Read the model definition and answer for the solid it produces. Units are mm, in the model's axes. Give positions to 0.01 mm unless a question says otherwise; leave off trailing zeros. Write each loop counter-clockwise with the first axis right and the second up, starting at its lowest first coordinate (ties: lowest second). Pieces come first, ordered by that corner, then holes. Notation, with made-up numbers: M 58,-17 L 74,-17 A22 ccw 74,22 Z; hole C 25,33.5 d4. An arc over 180 degrees is marked long. Use a Markdown table: item, result. Add a question column.
Item 1: The mould has two halves that part along X. Classify faces 1 (the cylindrical face through (0.86, -3.874, -64.389)), 2 (the conical face through (-4.16, -18.75, -61.76)), 3 (the flat face through (-0.3, 4.3, 0)): pulls with the +X half, pulls with the -X half, needs draft (parallel to the pull), parting line crosses it, or undercut.
Item 2: A cutting plane is placed at A-A on z = -37. Determine the outline of the cut face in (x, y).
Item 3: Given P1, Ø5, axis at x = -15, z = -84.5, coming from the -Y side; P2, Ø1, axis at x = -11, y = 14, coming from the -Z side; P3, Ø10, axis at x = 11, z = -23, coming from the +Y side; P4, Ø5, axis at x = 0, y = 0, coming from the -Z side, each flat-ended and moving along its own axis, determine where each tip first touches the part or whether it passes through.
Item 4: Consider probe 1 along Z at (x, y) = (-12, -10); probe 2 along Y at (x, z) = (0, -96.5); probe 3 along Y at (x, z) = (0, -28). Determine where each line is inside the solid, lowest interval first. Write a range as [from, to].
Item 5: A cutting plane is placed at B-B on z = -118.5. Determine the outline of the cut face in (x, y).
from build123d import *

# Parameters (mm, degrees)
F0_R = 18.034
F2_R = 20.447
F4_R = 5.08
F6_D = 7.9375


with BuildPart() as f3:
    # F0 (on Top) → F3 section 0
    with BuildSketch(Plane.XY):
        Circle(F0_R)
    # F2 (on offset) → F3 section 1
    with BuildSketch(Plane.XY.offset(-127)):
        Circle(F2_R)
    loft()

    # F4
    f4_edges = [f3.edges().sort_by_distance(p)[0] for p in [
        (-20.447, 0, -127),
    ]]
    fillet(f4_edges, radius=F4_R)

    # F6 (through all)
    with Locations(Plane.XY):
        with Locations((0, 0)):
            Hole(F6_D / 2)


solid = f3.part
Filled in:
| question | item | result |
|---|---|---|
| 1 | face 1 | undercut |
| 1 | face 2 | parting line crosses it |
| 1 | face 3 | needs draft |
| 2 | outline | C 0,0 d37.47; hole C 0,0 d7.94 |
| 3 | P1 | y = -15.15 |
| 3 | P2 | z = -126.57 |
| 3 | P3 | y = 17.47 |
| 3 | P4 | through |
| 4 | probe 1 | [-126.99, 0] |
| 4 | probe 2 | [-19.87, -3.97], [3.97, 19.87] |
| 4 | probe 3 | [-18.57, -3.97], [3.97, 18.57] |
| 5 | outline | C 0,0 d40.57; hole C 0,0 d7.94 |
